Source: CAD feature listing. Evaluate the final solid. Frame: model axes, mm. Face numbers are marked on the shaded views. Give positions to 0.01 mm unless a question says otherwise; leave off trailing zeros. Loops run counter-clockwise (first coordinate to the right, second up) from the corner with the lowest first, then second, coordinate; pieces in that order, holes last. Notation, with made-up numbers: M -7.75,-25 L 16.25,-25 A16 cw 16.25,-1 Z; hole C 2.25,31 d9. An arc over 180 degrees is marked long. Put each result on its own line as item: value.
from build123d import *

# Parameters (mm, degrees)
SKETCH1_R           = 7.5
BOSS_EXTRUDE1_DEPTH = 5
SKETCH2_R           = 5
CUT_EXTRUDE1_DEPTH  = 2.5
CHAMFER1_SIZE       = 2.5
SKETCH3_R           = 2.4
CUT_EXTRUDE2_DEPTH  = 2.5


with BuildPart() as part:
    # Sketch1 → Boss-Extrude1 (new body)
    with BuildSketch(Plane.XY):
        Circle(SKETCH1_R)
    extrude(amount=BOSS_EXTRUDE1_DEPTH)

    # Sketch2 → Cut-Extrude1 (cut)
    with BuildSketch(Plane.XY.offset(5)):
        Circle(SKETCH2_R)
    extrude(amount=-CUT_EXTRUDE1_DEPTH, mode=Mode.SUBTRACT)

    # Chamfer1
    chamfer1_edges = [part.edges().sort_by_distance(p)[0] for p in [
        (-7.5, 0, 0),
    ]]
    chamfer(chamfer1_edges, length=CHAMFER1_SIZE)

    # Sketch3 → Cut-Extrude2 (cut)
    with BuildSketch(Plane.XY.offset(2.5)):
        Circle(SKETCH3_R)
    extrude(amount=-CUT_EXTRUDE2_DEPTH, mode=Mode.SUBTRACT)


solid = part.part
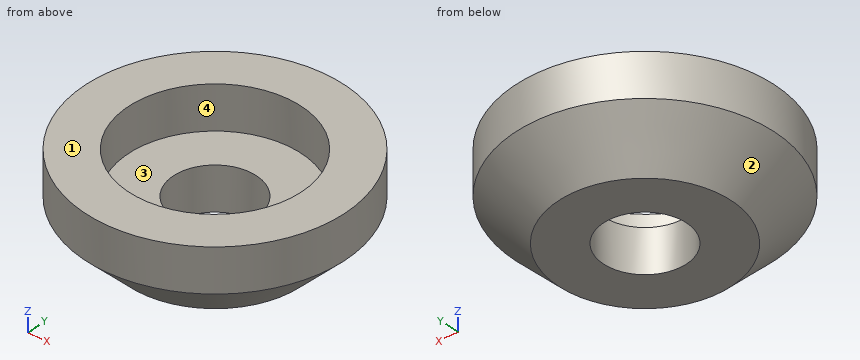
1. Contact query for flat-ended pins moving along their axis: P1, Ø3, axis at x = -2.5, z = 2, coming from the -Y side; P2, Ø1.5, axis at x = -5.5, z = 4, coming from the +Y side; P3, Ø9, axis at x = 0, y = 0, coming from the +Z side. Output: stop coordinate, or through.
Found:
P1: y = -7.42
P2: y = 5.8
P3: z = 2.5
2. Material intervals for line 1 (Y direction, x = 0, z = 4.4); line 2 (Y direction, x = 0, z = 0.7); line 3 (X direction, y = -1.25, z = 2.9), sorted ascending. Write a range as from..to.
Found:
line 1: -7.5..-5, 5..7.5
line 2: -5.7..-2.4, 2.4..5.7
line 3: -7.4..-4.84, 4.84..7.4
3. Draft query along X for the marked faces 1, 2, 3 and 4. Return one class per face: pulls with the +X half, pulls with the -X half, needs draft (parallel to the pull), parting line crosses it, or undercut.
Found:
face 1: needs draft
face 2: parting line crosses it
face 3: undercut
face 4: undercut
4. Section query A-A (y = 0). Output: boundary loops of the cut face in (x, z), plus the area to 4 significant figures.
Found:
outline: M -7.5,2.5 L -5,0 L -2.4,0 L -2.4,2.5 L -5,2.5 L -5,5 L -7.5,5 Z; M 2.4,0 L 5,0 L 7.5,2.5 L 7.5,5 L 5,5 L 5,2.5 L 2.4,2.5 Z
area: 31.75 mm^2
5. Section query C-C (z = 0.45). Output: boundary loops of the cut face in (x, y).
Found:
outline: C 0,0 d10.9; hole C 0,0 d4.8
6. Section query D-D (z = 3.75). Output: boundary loops of the cut face in (x, y).
Found:
outline: C 0,0 d15; hole C 0,0 d10
